Could you check a few things on this drawing? It's one solid part, dimensions in mm from its lowest x, y, z. A direction names the side the tool comes from. Give positions to 0.01 mm unless a question says otherwise; leave off trailing zeros. Loops run counter-clockwise (first coordinate to the right, second up) from the corner with the lowest first, then second, coordinate; pieces in that order, holes last. Notation, with made-up numbers: (86.25, 8) - (122.25, 8) arc R4 cw to (122.25, 14) - close; hole circle Ø1 at (-7.5, 51). An arc over 180 degrees is marked (long way). Write each question's results on one line, items separated by ' | '. Start each with the question number.
(1) On a 3-axis mill with a long thin cutter (end or side, diameter ignored), from which of +Z, -Z, +X, -X, +Y, -Y can I reach the whole of each face in a straight line? I mean the marked faces 4, 5 and 6. Say none if no direction works.
(2) Suppose I cut it at B-B (x = 14.5). Please give me the cut outline in (y, z), and give its area (3 significant figures).
(3) If we mould it in two halves opening along Z, with no side actions, what happens to the marked faces 1, 2 and 3? For each: released by +Z, released by -Z, zero draft, split by the parting line, or undercut.
(4) For pin 1 (3 mm diameter, centred on x = 10, z = 5, fed in from -Y); pin 2 (1 mm diameter, centred on x = 4.5, y = 1.5, fed in from -Z); pin 3 (0.7 mm diameter, centred on y = 3.5, z = 3, fed in from -X), each with a flat end and sliding along its axis, tell me the tip position at first contact or that it passes through.
(5) I need wall thicknesses on line 1 (X direction, y = 2.75, z = 3); line 2 (X direction, y = 5.5, z = 2); line 3 (Z direction, x = 1.25, y = 3.5). Which ranges of each line are inside material? Lowest first, please.
(6) Suppose I cut it at A-A (x = 12.5). Please give me the cut outline in (y, z).
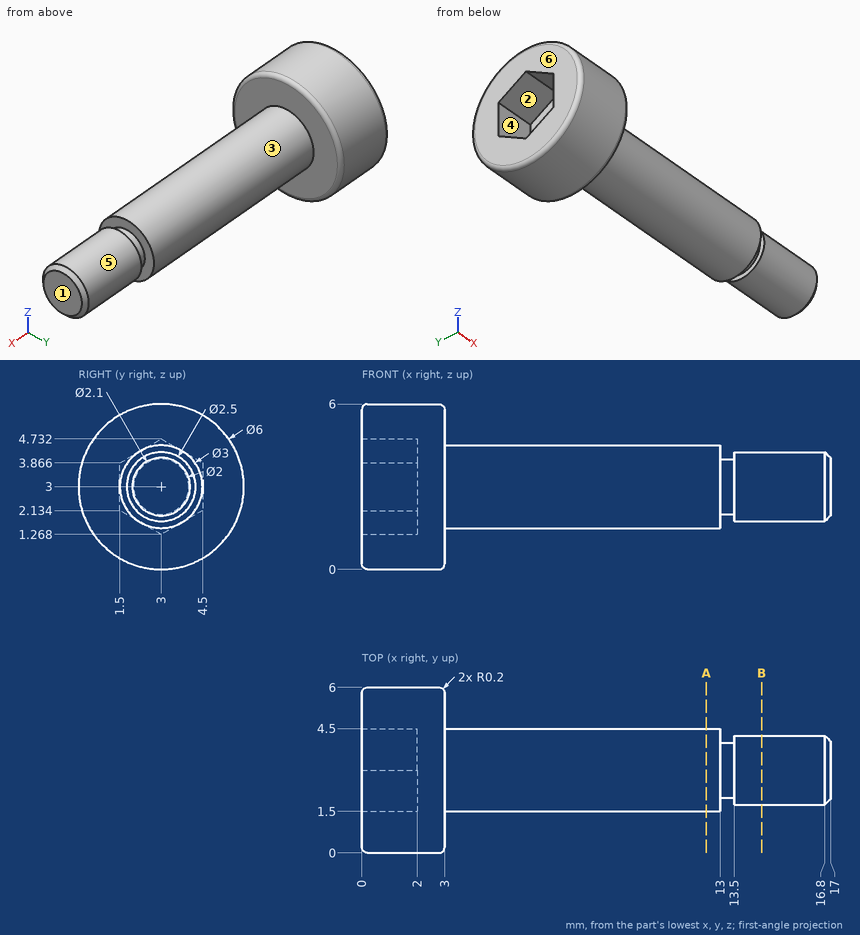
Output values:
1) face 4: -X | face 5: +X | face 6: +Z, -Z, -X, +Y, -Y
2) outline: circle Ø2.5 at (3, 3) | area: 4.91 mm2
3) face 1: zero draft | face 2: undercut | face 3: split by the parting line
4) pin 1: y = 1.59 | pin 2: z = 1.88 | pin 3: x = 2
5) line 1: 2 to 17 | line 2: 0 to 3 | line 3: 0.04 to 1.56, 4.44 to 5.96
6) outline: circle Ø3 at (3, 3)
